from build123d import *

# Parameters (mm, degrees)
EXTRUDE_1_DEPTH     = 70
SKETCH_3_W          = 91.211474189
SKETCH_3_H          = 70
EXTRUDE_3_DEPTH     = 20
SKETCH_7_R          = 37.5
CUT_EXTRUDE_1_DEPTH = 25
EXTRUDE_5_DEPTH     = 15


with BuildPart() as part:
    # 草图1 → 凸台-拉伸1 (new body)
    with BuildSketch(Plane.XY):
        Polygon((-88.329382669, -40.492222209), (2.88209152, -40.492222209), (2.88209152, 32.860075705), (-7.271573344, 79.507777791), (-8.937829763, 79.507777791), align=None)
    extrude(amount=EXTRUDE_1_DEPTH)

    # 草图3 → 凸台-拉伸3 (add)
    with BuildSketch(Plane.XZ.offset(40.492222209)):
        with Locations((-42.723645575, 35)):
            Rectangle(SKETCH_3_W, SKETCH_3_H)
    extrude(amount=EXTRUDE_3_DEPTH)

    # 草图7 → 切除-拉伸1 (cut)
    with BuildSketch(Plane.XY.offset(70)):
        with Locations((-22.66790848, -28.773433698)):
            Circle(SKETCH_7_R)
    extrude(amount=-CUT_EXTRUDE_1_DEPTH, mode=Mode.SUBTRACT)

    # 草图10 → 凸台-拉伸5 (add)
    with BuildSketch(Plane.XZ.offset(60.492222209)):
        Polygon((-88.329382669, 70), (-88.329382669, 0), (2.88209152, 0), (2.88209152, 70), (-2.663697539, 70), (-2.663697539, 45), (-42.672119422, 45), (-42.672119422, 70), align=None)
    extrude(amount=EXTRUDE_5_DEPTH)


solid = part.part
Check sheet for the modelled part. Datum: model origin and axes. Units: mm. A direction names the side the tool comes from. Round coordinates to 2 decimals unless told otherwise and drop trailing zeros. Loops run counter-clockwise (first coordinate to the right, second up) from the corner with the lowest first, then second, coordinate; pieces in that order, holes last. Notation, with made-up numbers: (40, 49) - (57, 49) arc R34 ccw to (57, 80) - close; hole circle Ø4 at (78, 43.25). An arc over 180 degrees is marked (long way). Answer as CSV lines item,"result". Start each with the question number.
Item 1: Section check C-C (x = -17). Record the boundary of the cut face in (y, z).
Item 2: Section check D-D (y = 57). Record the boundary of the cut face in (x, z), and give its area (3 significant figures).
Item 3: Depth check by flat-ended pin: P1, Ø2, axis at x = -40, z = 48, coming from the +Y side; P2, Ø10, axis at x = -70, z = 19.5, coming from the +Y side; P3, Ø3, axis at x = -48, z = 37.5, coming from the +Y side. Enter the tip coordinate at first touch or a pass-through.
Item 4: Scan lines: line 1 (Z direction, x = -5.5, y = -5); line 2 (Y direction, x = -25, z = 25.5); line 3 (Y direction, x = -50.5, z = 12). Record each from-to range of solid material in increasing order. Write a range as [from, to].
Item 5: Section check B-B (z = 4). Record the boundary of the cut face in (x, y).
Item 6: Set-up check for faces 1 (the cylindrical face through (0.17, -58.517, 57.675)), 2 (the flat face through (-43, -75.492, 28)), 3 (the flat face through (-42.672, -68, 57)): record each of +Z, -Z, +X, -X, +Y, -Y from which the full face is reachable in a straight line by a thin tool's end or side.
Item 7: Release check for a two-part mould opening along X. For faces 4 (the flat face through (-46, 2, 70)), 5 (the flat face through (2.882, -21, 27)), 6 (the cylindrical face through (-51.84, -5.21, 57.68)) record: +X half, -X half, draft (parallel to the pull), parting line (faces both ways), or undercut.
Item 8: Section check A-A (z = 62.5). Record the boundary of the cut face in (x, y), and give its area (3 significant figures).
Report:
1,outline,"(-75.49, 0) - (67.32, 0) - (67.32, 70) - (8.3, 70) - (8.3, 45) - (-75.49, 45) - close"
2,outline,"(-23.83, 0) - (-2.37, 0) - (-2.37, 70) - (-23.83, 70) - close"
2,area,"1,500 mm2"
3,P1,"stops at y = 34.07"
3,P2,"stops at y = -5.23"
3,P3,"stops at y = 22.73"
4,line 1,"z = [0, 45]"
4,line 2,"y = [-75.49, 55.23]"
4,line 3,"y = [-75.49, 16.69]"
5,outline,"(-88.33, -75.49) - (2.88, -75.49) - (2.88, 32.86) - (-7.27, 79.51) - (-8.94, 79.51) - (-88.33, -40.49) - close"
6,face 1,"+Z"
6,face 2,"+Z, -Z, +X, -X, -Y"
6,face 3,"+Z, -Y"
7,face 4,"draft"
7,face 5,"+X half"
7,face 6,"undercut"
8,outline,"(-88.33, -75.49) - (-42.67, -75.49) - (-42.67, -60.49) arc R37.5 cw (long way) to (2.88, -1.32) - (2.88, 32.86) - (-7.27, 79.51) - (-8.94, 79.51) - (-88.33, -40.49) - close; (-2.66, -75.49) - (2.88, -75.49) - (2.88, -56.22) arc R37.5 cw to (-2.66, -60.49) - close"
8,area,"4,730 mm2"
